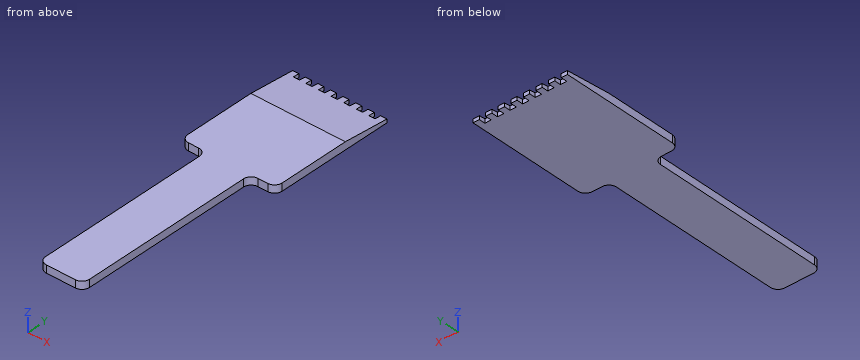
from build123d import *

# Parameters (mm, degrees)
F1_DEPTH = 3
F3_DEPTH = 65


with BuildPart() as f1:
    # F0 (on Top) → F1 (new body)
    with BuildSketch(Plane.XY):
        with BuildLine():
            Line((-17.5, 75), (-20, 75))
            Line((-20, 75), (-20, 72.5))
            Line((-20, 72.5), (-20, 28))
            ThreePointArc((-20, 28), (-19.1213203436, 25.8786796564), (-17, 25))
            Line((-17, 25), (-13, 25))
            ThreePointArc((-13, 25), (-10.8786796564, 24.1213203436), (-10, 22))
            Line((-10, 22), (-10, -47))
            ThreePointArc((-10, -47), (-9.1213203436, -49.1213203436), (-7, -50))
            Line((-7, -50), (-1.25, -50))
            Line((-1.25, -50), (4.5, -50))
            ThreePointArc((4.5, -50), (6.6213203436, -49.1213203436), (7.5, -47))
            Line((7.5, -47), (7.5, 22))
            ThreePointArc((7.5, 22), (8.3786796564, 24.1213203436), (10.5, 25))
            Line((10.5, 25), (14.5, 25))
            ThreePointArc((14.5, 25), (16.6213203436, 25.8786796564), (17.5, 28))
            Line((17.5, 28), (17.5, 75))
            Line((17.5, 75), (15, 75))
            Line((15, 75), (15, 72.4972039461))
            Line((15, 72.4972039461), (12.5, 72.4972039461))
            Line((12.5, 72.4972039461), (12.5, 75))
            Line((12.5, 75), (10, 75))
            Line((10, 75), (10, 72.4972039461))
            Line((10, 72.4972039461), (7.5, 72.4972039461))
            Line((7.5, 72.4972039461), (7.5, 75))
            Line((7.5, 75), (5, 75))
            Line((5, 75), (5, 72.4972039461))
            Line((5, 72.4972039461), (2.5, 72.4972039461))
            Line((2.5, 72.4972039461), (2.5, 75))
            Line((2.5, 75), (0, 75))
            Line((0, 75), (0, 72.4972039461))
            Line((0, 72.4972039461), (-1.25, 72.4972039461))
            Line((-1.25, 72.4972039461), (-2.5, 72.4972039461))
            Line((-2.5, 72.4972039461), (-2.5, 75))
            Line((-2.5, 75), (-5, 75))
            Line((-5, 75), (-5, 72.4972039461))
            Line((-5, 72.4972039461), (-7.5, 72.4972039461))
            Line((-7.5, 72.4972039461), (-7.5, 75))
            Line((-7.5, 75), (-10, 75))
            Line((-10, 75), (-10, 72.4972039461))
            Line((-10, 72.4972039461), (-12.5, 72.4972039461))
            Line((-12.5, 72.4972039461), (-12.5, 75))
            Line((-12.5, 75), (-15, 75))
            Line((-15, 75), (-15, 72.4972039461))
            Line((-15, 72.4972039461), (-17.5, 72.4972039461))
            Line((-17.5, 72.4972039461), (-17.5, 72.5))
            Line((-17.5, 72.5), (-17.5, 75))
        make_face()
    extrude(amount=F1_DEPTH)

    # F2 (on face) → F3 (cut)
    with BuildSketch(Plane.YZ.offset(17.5)):
        Polygon((75, 1.402389338), (78.919917345, 1.0673716897), (79.0749490261, 6.6061792895), (41.3183644414, 4.2810067534), (56.3069497208, 3), (75, 3), align=None)
        Polygon((56.3069497208, 3), (75, 1.402389338), (75, 3), align=None)
    extrude(amount=-F3_DEPTH, mode=Mode.SUBTRACT)


solid = f1.part
The model under review builds one solid part; all positions refer to its coordinate system, in mm. Give positions to 0.01 mm unless a question says otherwise; leave off trailing zeros. Write each loop counter-clockwise with the first axis right and the second up, starting at its lowest first coordinate (ties: lowest second). Pieces come first, ordered by that corner, then holes. Notation, with made-up numbers: M 57,52 L 93,52 A22 cw 93,77 Z; hole C 62,-5 d4. An arc over 180 degrees is marked long. One line per question, with ' | ' between items. Start each with the question number.
Item 1: We need section B-B on y = 13.5. Write out the cut boundary in (x, z).
Item 2: Wall thickness on line 1 (X direction, y = -32.5, z = 1.5); line 2 (Y direction, x = -7, z = 0.45); line 3 (Y direction, x = 11, z = 0.7): over which ranges is each line inside the solid? List them lowest first. Write a range as from..to.
Item 3: We need section C-C on y = 59.5. Write out the cut boundary in (x, z), plus the area to 3 significant figures.
Item 4: For pin 1 (3 mm diameter, centred on x = 7, y = 9, fed in from -Z); pin 2 (0.5 mm diameter, centred on x = 4, z = 0.5, fed in from +Y), all flat-tipped, find the tip position at first contact; note any pin that passes through.
Item 5: We need section A-A on z = 2.35. Write out the cut boundary in (x, y), plus the area to 3 significant figures.
Results found:
1) outline: M -10,0 L 7.5,0 L 7.5,3 L -10,3 Z
2) line 1: x = -10..7.5 | line 2: y = -50..72.5 | line 3: y = 25..75
3) outline: M -20,0 L 17.5,0 L 17.5,2.73 L -20,2.73 Z | area: 102 mm2
4) pin 1: stops at z = 0 | pin 2: stops at y = 72.5
5) outline: M -20,28 A3 ccw -17,25 L -13,25 A3 cw -10,22 L -10,-47 A3 ccw -7,-50 L 4.5,-50 A3 ccw 7.5,-47 L 7.5,22 A3 cw 10.5,25 L 14.5,25 A3 ccw 17.5,28 L 17.5,63.91 L -20,63.91 Z | area: 2,770 mm2
